Autodesk Inventor part; units mm, degrees
ref_plane "YZ Plane" through (0, 0, 0) normal (1, 0, 0) x (0, 1, 0)
ref_plane "XZ Plane" through (0, 0, 0) normal (0, 1, 0) x (-1, 0, 0)
ref_plane "XY Plane" through (0, 0, 0) normal (0, 0, 1) x (1, 0, 0)
sketch "Sketch1" plane through (0, 0, 0) normal (0, 0, 1) x (1, 0, 0)
  circle A0 centre (0, 0) radius 29
  circle A1 centre (0, 0) radius 60.5
  line L0 (-40.5, 60.5) -> (40.5, 60.5)
  line L1 (60.5, 40.5) -> (60.5, -40.5)
  line L2 (40.5, -60.5) -> (-40.5, -60.5)
  line L3 (-60.5, -40.5) -> (-60.5, 40.5)
  arc A2 (-40.5, 60.5) -> (-60.5, 40.5) centre (-40.5, 40.5) ccw
  arc A3 (60.5, 40.5) -> (40.5, 60.5) centre (40.5, 40.5) ccw
  arc A4 (40.5, -60.5) -> (60.5, -40.5) centre (40.5, -40.5) ccw
  arc A5 (-60.5, -40.5) -> (-40.5, -60.5) centre (-40.5, -40.5) ccw
  dimension "d0" = 58
  dimension "d1" = 121
  dimension "d2" = 20
extrude "Extrusion1" add sketch "Sketch1" along normal blind 1
sketch "Sketch2" plane through (0, 0, 1) normal (0, 0, 1) x (1, 0, 0)
  circle A0 centre (-48.4865, -48.5066) radius 2.65
  circle A1 centre (-37.2683, -53.25) radius 2.15
  circle A2 centre (-53.2329, -37.2897) radius 2.15
  circle A3 centre (-53.2431, 37.2752) radius 2.15
  circle A4 centre (-48.4997, 48.4934) radius 2.65
  circle A5 centre (-37.2829, 53.2398) radius 2.15
  circle A6 centre (37.2821, 53.25) radius 2.15
  circle A7 centre (48.5003, 48.5066) radius 2.65
  circle A8 centre (53.2467, 37.2897) radius 2.15
  circle A9 centre (53.2569, -37.2752) radius 2.15
  circle A10 centre (48.5135, -48.4934) radius 2.65
  circle A11 centre (37.2966, -53.2398) radius 2.15
  point P0 (0, 0)
extrude "Extrusion2" cut sketch "Sketch2" against normal through all
sketch "Sketch3" plane through (0, 0, 0) normal (0, 0, -1) x (-1, 0, 0)
  circle A0 centre (-0.0069, 0) radius 43
  point P0 (0, 0)
extrude "Extrusion3" cut sketch "Sketch3" against normal through all
properties part number "stator_mount_02_left_p" material "PC/ABS Plastic"
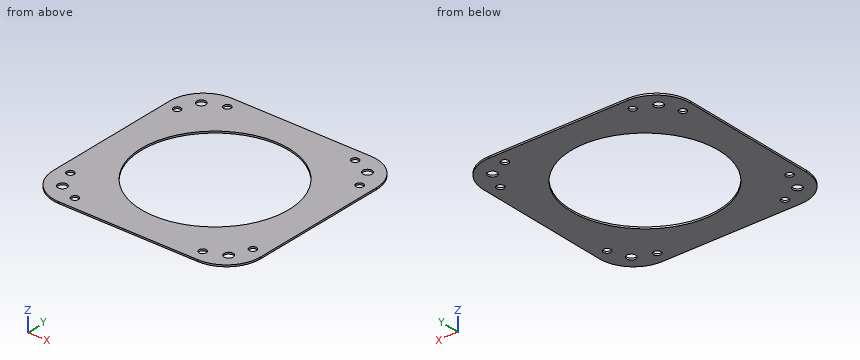
Geometry: final body of the model. Coordinates: model frame, mm. Round coordinates to 2 decimals unless told otherwise and drop trailing zeros. Loops run counter-clockwise (first coordinate to the right, second up) from the corner with the lowest first, then second, coordinate; pieces in that order, holes last.
Item 1: Line query: L1, parallel to Y at x = -35.5, z = 0.8; L2, parallel to Y at x = -49.5, z = 0.45; L3, parallel to X at y = -37.5, z = 0.5. Output: solid intervals per line, ascending.
Checked values:
L1: y = -60.5 to -54.47, -52.03 to -24.25, 24.25 to 52.04, 54.44 to 60.5
L2: y = -58.36 to -50.96, -46.06 to 46.04, 50.95 to 58.36
L3: x = -60.5 to -55.37, -51.09 to -21.03, 21.05 to 51.12, 55.4 to 60.5
Item 2: Contact query for a flat-ended pin moving along its axis: P1, Ø4, axis at x = 48.51, y = -48.49, coming from the -Z side. Output: stop coordinate, or through.
Checked values:
P1: passes through
Item 3: Section B-B, the plane x = -24. Output: boundary loops of the cut face in (y, z), plus the area to 3 significant figures.
Checked values:
outline: (-60.5, 0) - (-35.67, 0) - (-35.67, 1) - (-60.5, 1) - close; (35.67, 0) - (60.5, 0) - (60.5, 1) - (35.67, 1) - close
area: 49.7 mm2
Item 4: Section C-C, the plane z = 0.3. State how many separate pieces and enclosed holes the cut face has, plus the area to 3 significant figures.
Checked values:
separate pieces: 1
enclosed holes: 13
area: 8,280 mm2
Item 5: Section A-A, the plane y = 0. Output: boundary loops of the cut face in (x, z).
Checked values:
outline: (-60.5, 0) - (-42.99, 0) - (-42.99, 1) - (-60.5, 1) - close; (43.01, 0) - (60.5, 0) - (60.5, 1) - (43.01, 1) - close
